Could you check a few things on this model? Use its own coordinates, in mm. A direction names the side the tool comes from. Give positions to 0.01 mm unless a question says otherwise; leave off trailing zeros. Write each loop counter-clockwise with the first axis right and the second up, starting at its lowest first coordinate (ties: lowest second). Pieces come first, ordered by that corner, then holes. Notation, with made-up numbers: (86.5, -27.75) - (129.5, -27.75) arc R5 ccw to (129.5, -18.75) - close; hole circle Ø10 at (-25.5, 65.5). An arc over 180 degrees is marked (long way). Use one line per item in the form item = value.
```python
from build123d import *

# Parameters (mm, degrees)
F0_W        = 25.4
F0_H        = 25.4
F1_DEPTH    = 2
F2_W        = 17
F2_H        = 15
F3_DEPTH    = 1.905
F4_R        = 3.25
F5_DEPTH    = 2.6162
F7_D        = 2
F7_DEPTH    = 12.7
F7_TIP      = 0.600860619
F10_D       = 1.5
F10_ON_F8_D = 1.5


with BuildPart() as f1:
    # F0 (on Top) → F1 (new body)
    with BuildSketch(Plane.XY):
        Rectangle(F0_W, F0_H)
    extrude(amount=F1_DEPTH)

    # F2 (on Front) → F3 (join, symmetric)
    with BuildSketch(Plane.XZ):
        with Locations((0, 7.5)):
            Rectangle(F2_W, F2_H)
    extrude(amount=F3_DEPTH, both=True)

    # F4 (on Front) → F5 (cut, symmetric)
    with BuildSketch(Plane.XZ):
        with Locations((0, 15)):
            Circle(F4_R)
    extrude(amount=F5_DEPTH, both=True, mode=Mode.SUBTRACT)

    # F7
    with Locations(Plane.XY.offset(15)):
        with Locations((5.875, 0), (-5.875, 0)):
            Hole(F7_D / 2, depth=F7_DEPTH)
            with Locations((0, 0, -(F7_DEPTH + F7_TIP / 2))):  # 118° drill point
                Cone(0, F7_D / 2, F7_TIP, mode=Mode.SUBTRACT)

    # F10 (through all)
    with Locations(Plane.YZ.offset(8.5)):
        with Locations((0, 13.5882580653)):
            Hole(F10_D / 2)

    # F10 on F8 (through all)
    with Locations(Plane(origin=(-8.5, 0, 0), x_dir=(0, -1, 0), z_dir=(-1, 0, 0))):
        with Locations((0, 13.4879248217)):
            Hole(F10_ON_F8_D / 2)


solid = f1.part
```
1. Imagine slicing it at A-A, the plane z = 7.5. List the corners of the cut face in (x, y) for me (3 decimals).
Response values:
outline = (-8.5, -1.905) - (8.5, -1.905) - (8.5, 1.905) - (-8.5, 1.905) - close; hole circle Ø2 at (-5.875, 0); hole circle Ø2 at (5.875, 0)
2. If I drill on line 1 (X direction, y = 0, z = 3.75) (3 decimals); line 2 (Y direction, x = -6, z = 3) (3 decimals); line 3 (Z direction, x = 6, y = 9.25), over which ranges is the centre line in solid material (lowest first)? Write a range as from..to.
Response values:
line_1 = -8.5..-6.875, -4.875..4.875, 6.875..8.5
line_2 = -1.905..-0.992, 0.992..1.905
line_3 = 0..2
3. Imagine slicing it at C-C, the plane x = -7.5. List the corners of the cut face in (y, z) for me (3 decimals).
Response values:
outline = (-12.7, 0) - (12.7, 0) - (12.7, 2) - (1.905, 2) - (1.905, 15) - (-1.905, 15) - (-1.905, 2) - (-12.7, 2) - close; hole (-0.748, 13.538) arc R0.75 ccw (long way) to (0.748, 13.538) arc R0.75 ccw (long way) to start
4. Imagine slicing it at D-D, the plane y = -3.5. List the corners of the cut face in (x, z) for me.
Response values:
outline = (-12.7, 0) - (12.7, 0) - (12.7, 2) - (-12.7, 2) - close
5. If we mould it in two halves opening along Y, with no side actions, what happens to faces 4 (the face through (5.702, 0.008, 1.803)), 5 (the face through (12.7, 0, 1)), 6 (the face through (0, -12.7, 1))? For each: pulls with the +Y half, pulls with the -Y half, needs draft (parallel to the pull), parting line crosses it, or undercut.
Response values:
face_4 = undercut
face_5 = needs draft
face_6 = pulls with the -Y half
6. For pin 1 (5 mm diameter, centred on y = 4, z = 7, fed in from -X); pin 2 (4 mm diameter, centred on x = 3.5, z = 10.5, fed in from -Y) (3 decimals); pin 3 (4 mm diameter, centred on y = -0.5, z = 9, fed in from +X); pin 4 (1 mm diameter, centred on x = 7.5, y = -5.5, fed in from -Z), each with a flat end and sliding along its axis, tell me the tip position at first contact or that it passes through.
Response values:
pin_1 = -8.5
pin_2 = -1.905
pin_3 = 8.5
pin_4 = 0
7. Which directions (+Z, -Z, +X, -X, +Y, -Y) give clear straight access to the entire face, cutting with the end or side of a thin tool? Please do faces 1 (the face through (-3.75, -0.02, 12.74)), 2 (the face through (0, 1.905, 9)), 3 (the face through (0, -1.905, 9)).
Response values:
face_1 = +X, -X
face_2 = +Z, +X, -X, +Y
face_3 = +Z, +X, -X, -Y
8. Imagine slicing it at B-B, the plane x = 0. List the corners of the cut face in (y, z) for me (3 decimals), and give its area (3 significant figures).
Response values:
outline = (-12.7, 0) - (12.7, 0) - (12.7, 2) - (1.905, 2) - (1.905, 11.75) - (-1.905, 11.75) - (-1.905, 2) - (-12.7, 2) - close
area = 87.9 mm²
